Build history of the part. All positions in model axes, mm. A direction names the side the tool comes from. Give positions to 0.01 mm unless a question says otherwise; leave off trailing zeros. Order: outer loops, then holes, each group sorted by start corner. A loop starts at its lowest first (then second) coordinate and runs counter-clockwise, first axis right, second up. Notation, with made-up numbers: (60, 33.25) -> (101, 33.25) arc R10 cw to (101, 52.25) -> close; hole circle Ø7 at (-38, 46.25). An arc over 180 degrees is marked (long way). Write item = value, one per line. Start each with the question number.
from build123d import *

# Parameters (mm, degrees)
BOSS_EXTRUDE2_DEPTH = 200
FILLET2_R           = 17
SKETCH3_R           = 5.05
CUT_EXTRUDE1_DEPTH  = 200
SKETCH4_R           = 1.3
CUT_EXTRUDE3_DEPTH  = 35
SKETCH5_W           = 80
SKETCH5_H           = 38
SKETCH5_H_2         = 30
CUT_EXTRUDE4_DEPTH  = 21
FILLET3_R           = 8
SKETCH6_W           = 3
SKETCH6_H           = 32
CUT_EXTRUDE5_DEPTH  = 21
SKETCH8_W           = 30
SKETCH8_H           = 50
CUT_EXTRUDE6_DEPTH  = 21
FILLET4_R           = 6
SKETCH9_W           = 30
SKETCH9_H           = 50
CUT_EXTRUDE7_DEPTH  = 21
FILLET5_R           = 6
SKETCH10_W          = 60
SKETCH10_H          = 2.25
BOSS_EXTRUDE3_DEPTH = 5
CHAMFER1_SIZE       = 5
CHAMFER2_SIZE       = 5
FILLET6_R           = 1
SKETCH11_W          = 60
SKETCH11_H          = 2.25
BOSS_EXTRUDE4_DEPTH = 5
CHAMFER3_SIZE       = 5
FILLET7_R           = 1
SKETCH12_R          = 1.6
CUT_EXTRUDE9_DEPTH  = 21
SKETCH13_R          = 3
CUT_EXTRUDE10_DEPTH = 2


with BuildPart() as part:
    # Sketch1 → Boss-Extrude2 (new body)
    with BuildSketch(Plane(origin=(0, 0, 0), x_dir=(1, 0, 0), z_dir=(0, 1, 0))):
        Polygon((-67.942807508, 35.802956243), (72.381423465, 35.802956243), (54.719307979, -35.035919795), (-50.280692021, -35.035919795), align=None)
        Polygon((-45.280692021, -29.035919795), (49.719307979, -29.035919795), (64.389487431, 29.802956243), (-59.950871474, 29.802956243), align=None, mode=Mode.SUBTRACT)
    extrude(amount=BOSS_EXTRUDE2_DEPTH)

    # Fillet2
    fillet2_edges = [part.edges().sort_by_distance(p)[0] for p in [
        (64.389487431, 100, -29.802956243),
        (-59.950871474, 100, -29.802956243),
    ]]
    fillet(fillet2_edges, radius=FILLET2_R)

    # Sketch3 → Cut-Extrude1 (cut)
    with BuildSketch(Plane(origin=(0, 200, 0), x_dir=(1, 0, 0), z_dir=(0, 1, 0))):
        with Locations(Location((-58.192807508, 27.802956243, 0), (0, 0, 270))):
            Circle(SKETCH3_R)
        with Locations(Location((62.631423465, 27.802956243, 0), (0, 0, 270))):
            Circle(SKETCH3_R)
    extrude(amount=-CUT_EXTRUDE1_DEPTH, mode=Mode.SUBTRACT)

    # Sketch4 → Cut-Extrude3 (cut)
    with BuildSketch(Plane(origin=(0, 0, -35.802956243), x_dir=(-1, 0, 0), z_dir=(0, 0, -1))):
        with Locations((9.092807508, 60)):
            Circle(SKETCH4_R)
        with Locations((-13.527192492, 60)):
            Circle(SKETCH4_R)
        with Locations((9.092807508, 140)):
            Circle(SKETCH4_R)
        with Locations((-2.217192492, 140)):
            Circle(SKETCH4_R)
        with Locations((-13.527192492, 140)):
            Circle(SKETCH4_R)
        with Locations((-2.217192492, 60)):
            Circle(SKETCH4_R)
    extrude(amount=-CUT_EXTRUDE3_DEPTH, mode=Mode.SUBTRACT)

    # Sketch5 → Cut-Extrude4 (cut)
    with BuildSketch(Plane(origin=(0, 0, -35.802956243), x_dir=(-1, 0, 0), z_dir=(0, 0, -1))):
        with Locations((-2.217192492, 100)):
            Rectangle(SKETCH5_W, SKETCH5_H)
        with Locations((-2.217192492, 171)):
            Rectangle(SKETCH5_W, SKETCH5_H_2)
        with Locations((-2.217192492, 29)):
            Rectangle(SKETCH5_W, SKETCH5_H_2)
    extrude(amount=-CUT_EXTRUDE4_DEPTH, mode=Mode.SUBTRACT)

    # Fillet3
    fillet3_edges = [part.edges().sort_by_distance(p)[0] for p in [
        (-37.782807508, 186, -32.802956243),
        (-37.782807508, 156, -32.802956243),
        (42.217192492, 156, -32.802956243),
        (42.217192492, 186, -32.802956243),
        (-37.782807508, 119, -32.802956243),
        (-37.782807508, 81, -32.802956243),
        (42.217192492, 81, -32.802956243),
        (42.217192492, 119, -32.802956243),
        (-37.782807508, 44, -32.802956243),
        (-37.782807508, 14, -32.802956243),
        (42.217192492, 14, -32.802956243),
        (42.217192492, 44, -32.802956243),
    ]]
    fillet(fillet3_edges, radius=FILLET3_R)

    # Sketch6 → Cut-Extrude5 (cut)
    with BuildSketch(Plane.XY.offset(35.035919795)):
        with Locations((-40.780692021, 174)):
            Rectangle(SKETCH6_W, SKETCH6_H)
        with Locations((-40.780692021, 26)):
            Rectangle(SKETCH6_W, SKETCH6_H)
        with Locations((45.219307979, 26)):
            Rectangle(SKETCH6_W, SKETCH6_H)
        with Locations((45.219307979, 174)):
            Rectangle(SKETCH6_W, SKETCH6_H)
    extrude(amount=-CUT_EXTRUDE5_DEPTH, mode=Mode.SUBTRACT)

    # Sketch8 → Cut-Extrude6 (cut)
    with BuildSketch(Plane(origin=(59.740978631, 0, 14.89509889), x_dir=(0.24192189559966498, 0, -0.9702957262759973), z_dir=(0.9702957262759971, 0, 0.24192189559966495))):
        with Locations((7.250106602, 47)):
            Rectangle(SKETCH8_W, SKETCH8_H)
        with Locations((7.250106602, 153)):
            Rectangle(SKETCH8_W, SKETCH8_H)
    extrude(amount=-CUT_EXTRUDE6_DEPTH, mode=Mode.SUBTRACT)

    # Fillet4
    fillet4_edges = [part.edges().sort_by_distance(p)[0] for p in [
        (62.065874762, 72, -7.456502519),
        (62.065874762, 22, -7.456502519),
        (54.808217894, 22, 21.652369269),
        (54.808217894, 72, 21.652369269),
        (62.065874762, 178, -7.456502519),
        (62.065874762, 128, -7.456502519),
        (54.808217894, 128, 21.652369269),
        (54.808217894, 178, 21.652369269),
    ]]
    fillet(fillet4_edges, radius=FILLET4_R)

    # Sketch9 → Cut-Extrude7 (cut)
    with BuildSketch(Plane(origin=(-55.562138014, 0, 13.853196905), x_dir=(0.2419218955996648, 0, 0.9702957262759973), z_dir=(-0.9702957262759973, 0, 0.2419218955996648))):
        with Locations((-6.176308215, 47)):
            Rectangle(SKETCH9_W, SKETCH9_H)
        with Locations((-6.176308215, 153)):
            Rectangle(SKETCH9_W, SKETCH9_H)
    extrude(amount=-CUT_EXTRUDE7_DEPTH, mode=Mode.SUBTRACT)

    # Fillet5
    fillet5_edges = [part.edges().sort_by_distance(p)[0] for p in [
        (-50.369601937, 72, 21.652369269),
        (-50.369601937, 22, 21.652369269),
        (-57.627258805, 22, -7.456502519),
        (-57.627258805, 72, -7.456502519),
        (-57.627258805, 128, -7.456502519),
        (-57.627258805, 178, -7.456502519),
        (-50.369601937, 178, 21.652369269),
        (-50.369601937, 128, 21.652369269),
    ]]
    fillet(fillet5_edges, radius=FILLET5_R)

    # Sketch10 → Boss-Extrude3 (add)
    with BuildSketch(Plane(origin=(0, 0, 29.035919795), x_dir=(-1, 0, 0), z_dir=(0, 0, -1))):
        with Locations((-2.219307979, 1.125)):
            Rectangle(SKETCH10_W, SKETCH10_H)
    extrude(amount=BOSS_EXTRUDE3_DEPTH)

    # Chamfer1
    chamfer1_edges = [part.edges().sort_by_distance(p)[0] for p in [
        (32.219307979, 1.125, 24.035919795),
    ]]
    chamfer(chamfer1_edges, length=CHAMFER1_SIZE - 0.0001)  # a hair under: the kernel refuses the full size

    # Chamfer2
    chamfer2_edges = [part.edges().sort_by_distance(p)[0] for p in [
        (-27.780692021, 1.125, 24.035919795),
    ]]
    chamfer(chamfer2_edges, length=CHAMFER2_SIZE - 0.0001)  # a hair under: the kernel refuses the full size

    # Fillet6
    fillet6_edges = [part.edges().sort_by_distance(p)[0] for p in [
        (2.219307979, 2.25, 29.035919795),
    ]]
    fillet(fillet6_edges, radius=FILLET6_R)

    # Sketch11 → Boss-Extrude4 (add)
    with BuildSketch(Plane(origin=(0, 0, 29.035919795), x_dir=(-1, 0, 0), z_dir=(0, 0, -1))):
        with Locations((-2.219307979, 198.875)):
            Rectangle(SKETCH11_W, SKETCH11_H)
    extrude(amount=BOSS_EXTRUDE4_DEPTH)

    # Chamfer3
    chamfer3_edges = [part.edges().sort_by_distance(p)[0] for p in [
        (32.219307979, 198.875, 24.035919795),
        (-27.780692021, 198.875, 24.035919795),
    ]]
    chamfer(chamfer3_edges, length=CHAMFER3_SIZE - 0.0001)  # a hair under: the kernel refuses the full size

    # Fillet7
    fillet7_edges = [part.edges().sort_by_distance(p)[0] for p in [
        (2.219307979, 197.75, 29.035919795),
    ]]
    fillet(fillet7_edges, radius=FILLET7_R)

    # Sketch12 → Cut-Extrude9 (cut)
    with BuildSketch(Plane.XY.offset(35.035919795)):
        with Locations((27.219307979, 48.22)):
            Circle(SKETCH12_R)
        with Locations((-22.780692021, 48.22)):
            Circle(SKETCH12_R)
        with Locations((27.219307979, 151.78)):
            Circle(SKETCH12_R)
        with Locations((-22.780692021, 151.78)):
            Circle(SKETCH12_R)
    extrude(amount=-CUT_EXTRUDE9_DEPTH, mode=Mode.SUBTRACT)

    # Sketch13 → Cut-Extrude10 (cut)
    with BuildSketch(Plane(origin=(0, 0, 29.035919795), x_dir=(-1, 0, 0), z_dir=(0, 0, -1))):
        with Locations((-27.219307979, 48.22)):
            Circle(SKETCH13_R)
        with Locations((22.780692021, 48.22)):
            Circle(SKETCH13_R)
        with Locations((-27.219307979, 151.78)):
            Circle(SKETCH13_R)
        with Locations((22.780692021, 151.78)):
            Circle(SKETCH13_R)
    extrude(amount=-CUT_EXTRUDE10_DEPTH, mode=Mode.SUBTRACT)


solid = part.part
(1) Cut at D-D, the plane y = 104.5. Give the cut face in (x, z), plus the area to 3 significant figures.
(2) Cut at B-B, the plane x = 20.5. Give the cut face in (y, z), plus the area to 3 significant figures.
(3) Wall check: line 1 (Z direction, x = 10.5, y = 153); line 2 (X direction, y = 126, z = -24.5); line 3 (X direction, y = 140, z = -31.6). Give the ranges that are in metal, low to high. Write a range as [from, to].
(4) Mould opens along X. For faces 1 (the face through (-50.741, 70.196, 19.982)), 2 (the face through (39.81, 16.28, -32.76)), 3 (the face through (-57.67, 46.734, -7.446)), 4 (the face through (54.851, 152.734, 21.663)) say: released by +X, released by -X, zero draft, split by the parting line, or undercut.
(5) Cut at A-A, the plane y = 144. Give the cut face in (x, z), plus the area to 3 significant figures.
(6) Cut at C-C, the plane z = -26. Give the cut face in (x, y).
(7) 3-axis set-ups, long thin cutter, end or side, ignore diameter. For faces 5 (the face through (-25.316, 1.236, 26.571)), 6 (the face through (62.109, 152.734, -7.446)), 7 (the face through (3, 156, -33)), 8 (the face through (27.61, 154.754, 30.022)), 9 (the face through (55.2, 129.71, 19.89)): which of +Z, -Z, +X, -X, +Y, -Y reach the whole face in a straight line?
(8) Flat gauge pins, fed straight in: P1, Ø1.5, axis at y = 103, z = -23, coming from the +X side; P2, Ø5, axis at y = 171.5, z = -32.5, coming from the +X side; P3, Ø1.8, axis at y = 19, z = 33.5, coming from the +X side. Where does each tip first touch, or does it go through?
Results:
q1.outline = (-67.94, -35.8) -> (-37.78, -35.8) -> (-37.78, -29.8) -> (-38.19, -29.8) arc R17 cw to (-54.69, -8.69) -> (-45.28, 29.04) -> (49.72, 29.04) -> (59.13, -8.69) arc R17 cw to (42.63, -29.8) -> (42.22, -29.8) -> (42.22, -35.8) -> (72.38, -35.8) -> (54.72, 35.04) -> (-50.28, 35.04) -> close; hole circle Ø10.1 at (-58.19, -27.8); hole circle Ø10.1 at (62.63, -27.8)
q1.area = 1,810 mm2
q2.outline = (0, -35.8) -> (14, -35.8) -> (14, -29.8) -> (0, -29.8) -> close; (0, 24.04) -> (2.25, 24.04) -> (2.25, 28.04) arc R1 cw to (3.25, 29.04) -> (196.75, 29.04) arc R1 cw to (197.75, 28.04) -> (197.75, 24.04) -> (200, 24.04) -> (200, 35.04) -> (0, 35.04) -> close; (44, -35.8) -> (81, -35.8) -> (81, -29.8) -> (44, -29.8) -> close; (119, -35.8) -> (156, -35.8) -> (156, -29.8) -> (119, -29.8) -> close; (186, -35.8) -> (200, -35.8) -> (200, -29.8) -> (186, -29.8) -> close
q2.area = 1,830 mm2
q3.line_1 = [-35.8, -29.8], [29.04, 35.04]
q3.line_2 = [-65.12, -62.01], [-54.37, -50.53], [54.97, 58.81], [66.45, 69.56]
q3.line_3 = [-66.89, -61.52], [-54.86, -10.39], [-7.79, 0.92], [3.52, 12.23], [14.83, 59.3], [65.96, 71.33]
q4.face_1 = released by -X
q4.face_2 = undercut
q4.face_3 = undercut
q4.face_4 = released by +X
q5.outline = (-67.94, -35.8) -> (72.38, -35.8) -> (65.12, -6.69) -> (59.01, -8.22) -> (59.13, -8.69) arc R17 cw to (42.63, -29.8) -> (-38.19, -29.8) arc R17 cw to (-54.69, -8.69) -> (-54.57, -8.22) -> (-60.69, -6.69) -> close; (-53.43, 22.41) -> (-47.31, 20.89) -> (-45.28, 29.04) -> (49.72, 29.04) -> (51.75, 20.89) -> (57.87, 22.41) -> (54.72, 35.04) -> (-50.28, 35.04) -> close; hole circle Ø10.1 at (-58.19, -27.8); hole circle Ø10.1 at (62.63, -27.8)
q5.area = 1,910 mm2
q6.outline = (-65.5, 0) -> (-62.91, 0) -> (-62.91, 200) -> (-65.5, 200) -> close; (-53.48, 0) -> (-48.91, 0) -> (-48.91, 200) -> (-53.48, 200) -> close; (53.35, 0) -> (57.91, 0) -> (57.91, 200) -> (53.35, 200) -> close; (67.35, 0) -> (69.94, 0) -> (69.94, 200) -> (67.35, 200) -> close
q7.face_5 = +Y, -Y
q7.face_6 = +Z
q7.face_7 = -Z
q7.face_8 = none
q7.face_9 = +X
q8.P1 = 69.38
q8.P2 = 72.18
q8.P3 = 55.33
